Can you work these out from the model? Positions are in its coordinate system, mm. Face numbers are marked on the shaded views. Round coordinates to 2 decimals unless told otherwise and drop trailing zeros. Order: outer loops, then holes, each group sorted by start corner. A loop starts at its lowest first (then second) coordinate and runs counter-clockwise, first axis right, second up.
Q1. If I drill on line 1 (Y direction, x = -1, z = 0); line 2 (Z direction, x = 3.15, y = 0); line 3 (Y direction, x = -3.2, z = 0), over which ranges is the centre line in solid material (lowest first)?
Q2. Will these pins go through, and if not, where does the flat tip stop? P1, Ø4, axis at x = -2, y = 10, coming from the -Z side; P2, Ø2, axis at x = 0.5, z = 12, coming from the +Y side.
Q3. If we section it at C-C (x = 1.5): Please give me the cut outline in (y, z).
Q4. We'd pull the mould along Z, two halves only. Please class the marked faces 1, 2 and 3: pulls with the +Z half, pulls with the -Z half, needs draft (parallel to the pull), parting line crosses it, or undercut.
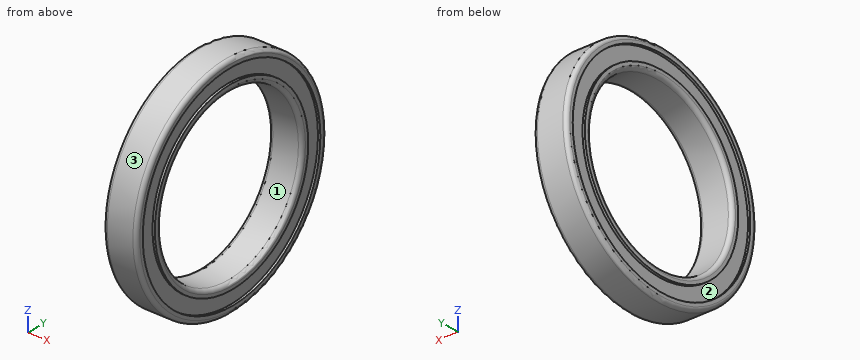
from build123d import *

# Parameters (mm, degrees)
FILLET_1_R = 0.8


with BuildPart() as part:
    # Эскиз1 → Повернуть1 (revolve)
    with BuildSketch(Plane.XY):
        Polygon((3.5, 17.5), (-3.5, 17.5), (-3.5, 19), (-3, 19), (-3, 22), (-3.5, 22), (-3.5, 23.5), (3.5, 23.5), (3.5, 22), (3, 22), (3, 19), (3.5, 19), align=None)
    revolve(axis=Axis((0, 0, 0), (-1, 0, 0)))

    # Скругление1
    fillet_1_edges = [part.edges().sort_by_distance(p)[0] for p in [
        (-3.5, -23.5, 0),
        (3.5, -23.5, 0),
        (3.5, -17.5, 0),
        (-3.5, -17.5, 0),
    ]]
    fillet(fillet_1_edges, radius=FILLET_1_R)


solid = part.part
Solution:
1. line 1: y = -23.5 to -17.5, 17.5 to 23.5
1. line 2: z = -23.36 to -22, -19 to -17.64, 17.64 to 19, 22 to 23.36
1. line 3: y = -23.32 to -22, -19 to -17.68, 17.68 to 19, 22 to 23.32
2. P1: stops at z = -22.1
2. P2: stops at y = 20.77
3. outline: circle Ø47 at (0, 0); hole circle Ø35 at (0, 0)
4. face 1: undercut
4. face 2: undercut
4. face 3: parting line crosses it
